```python
from build123d import *

# Parameters (mm, degrees)
SKETCH_1_R      = 1.5
EXTRUDE_1_DEPTH = 1.2
SKETCH_2_W      = 56.26507056
SKETCH_2_H      = 7.246466171
SKETCH_2_W_2    = 5.94694539
SKETCH_2_H_2    = 46.466862472
SKETCH_2_W_3    = 61.857792897
SKETCH_2_H_3    = 5.88577246
SKETCH_2_W_4    = 11.220508583
SKETCH_2_H_4    = 22.405589271
EXTRUDE_2_DEPTH = 9


with BuildPart() as part:
    # 草图1 → 凸台-拉伸1 (new body)
    with BuildSketch(Plane(origin=(0, 0, 0), x_dir=(1, 0, 0), z_dir=(0, 1, 0))):
        with BuildLine():
            Line((39.65, 36.5), (-39.65, 36.5))
            ThreePointArc((-39.65, 36.5), (-41.771320344, 35.621320344), (-42.65, 33.5))
            Line((-42.65, 33.5), (-42.65, -33.5))
            ThreePointArc((-42.65, -33.5), (-41.771320344, -35.621320344), (-39.65, -36.5))
            Line((-39.65, -36.5), (39.65, -36.5))
            ThreePointArc((39.65, -36.5), (41.771320344, -35.621320344), (42.65, -33.5))
            Line((42.65, -33.5), (42.65, 33.5))
            ThreePointArc((42.65, 33.5), (41.771320344, 35.621320344), (39.65, 36.5))
        make_face()
        with Locations(Location((39.65, -33.5, 0), (0, 0, 270))):
            Circle(SKETCH_1_R, mode=Mode.SUBTRACT)
        with Locations(Location((-39.65, -33.5, 0), (0, 0, 270))):
            Circle(SKETCH_1_R, mode=Mode.SUBTRACT)
        with Locations(Location((-39.65, 33.5, 0), (0, 0, 270))):
            Circle(SKETCH_1_R, mode=Mode.SUBTRACT)
        with Locations(Location((39.65, 33.5, 0), (0, 0, 270))):
            Circle(SKETCH_1_R, mode=Mode.SUBTRACT)
    extrude(amount=EXTRUDE_1_DEPTH)

    # 草图2 → 凸台-拉伸2 (add)
    with BuildSketch(Plane(origin=(0, 1.2, 0), x_dir=(1, 0, 0), z_dir=(0, 1, 0))):
        with Locations((3.299265125, -32.876766915)):
            Rectangle(SKETCH_2_W, SKETCH_2_H)
        with Locations((39.676527305, 1.231104757)):
            Rectangle(SKETCH_2_W_2, SKETCH_2_H_2)
        with Locations((-0.500594968, 33.55711377)):
            Rectangle(SKETCH_2_W_3, SKETCH_2_H_3)
        with Locations((-37.039745709, 3.646177151)):
            Rectangle(SKETCH_2_W_4, SKETCH_2_H_4)
    extrude(amount=EXTRUDE_2_DEPTH)


solid = part.part
```
Model file for the job. Use its own axes, mm. A direction names the side the tool comes from. Coordinates: 2 decimals unless noted, no trailing zeros. Loops run counter-clockwise (first coordinate to the right, second up) from the corner with the lowest first, then second, coordinate; pieces in that order, holes last. Notation, with made-up numbers: M 55,-14 L 93,-14 A21 ccw 93,-3 Z; hole C 1.25,36.5 d3. An arc over 180 degrees is marked long. Use CSV: the item, a comma, the result in double quotes. Start each with the question number.
1. Flat gauge pins, fed straight in: pin 1 (3 mm diameter, centred on x = 13, z = -0.5, fed in from +Y); pin 2 (6 mm diameter, centred on x = -33, y = 7.5, fed in from +Z); pin 3 (4.5 mm diameter, centred on y = 6, z = -33, fed in from -X). Where does each tip first touch, or does it go through?
2. Probe probe 1 along X at (y, z) = (0.95, -33.5); probe 2 along X at (y, z) = (4.25, -7); probe 3 along Z at (x, y) = (26, 8). List the from-to ranges inside material, lowest first. Write a range as [from, to].
3. Band-saw the part on A-A, the plane y = 3.75. List the corners of the cut face in (x, z), then the cut area to 3 significant figures.
4. Band-saw the part on D-D, the plane z = 26. List the corners of the cut face in (x, y).
5. Two-plate mould, pull along Z, no slides. Class faces 5 (the flat face through (-1, 6, -30.614)), 6 (the flat face through (-24.833, 6, 33)), 7 (the cylindrical face through (41.75, 0.59, 35.64)): pulls with the +Z half, pulls with the -Z half, needs draft (parallel to the pull), parting line crosses it, or undercut.
6. Band-saw the part on B-B, the plane z = -22. List the corners of the cut face in (x, y).
7. Tool access for faces 1 (the flat face through (3, 6, 29.254)), 2 (the flat face through (40, 6, 22.002)), 3 (the flat face through (30.428, 6, -34)), 4 (the flat face through (-37, 6, -14.849)): list every direction of +Z, -Z, +X, -X, +Y, -Y with a clear straight run to the whole face (end or side of a thin tool).
8. Band-saw the part on C-C, the plane x = -4. List the corners of the cut face in (y, z).
Entries:
1,pin 1,"stops at y = 1.2"
1,pin 2,"stops at z = 7.56"
1,pin 3,"stops at x = -31.43"
2,probe 1,"x = [-42.65, -41.15], [-38.15, 38.15], [41.15, 42.65]"
2,probe 2,"x = [-42.65, -31.43], [36.7, 42.65]"
2,probe 3,"z = [-36.5, -30.61], [29.25, 36.5]"
3,outline,"M -42.65,-14.85 L -31.43,-14.85 L -31.43,7.56 L -42.65,7.56 Z; M -31.43,-36.5 L 30.43,-36.5 L 30.43,-30.61 L -31.43,-30.61 Z; M -24.83,29.25 L 31.43,29.25 L 31.43,36.5 L -24.83,36.5 Z; M 36.7,-24.46 L 42.65,-24.46 L 42.65,22 L 36.7,22 Z"
3,area,"1,300 mm2"
4,outline,"M -42.65,0 L 42.65,0 L 42.65,1.2 L -42.65,1.2 Z"
5,face 5,"undercut"
5,face 6,"needs draft"
5,face 7,"pulls with the +Z half"
6,outline,"M -42.65,0 L 42.65,0 L 42.65,10.2 L 36.7,10.2 L 36.7,1.2 L -42.65,1.2 Z"
7,face 1,"+X, -X, +Y"
7,face 2,"+Z, +X, -X, +Y"
7,face 3,"-Z, +X, +Y"
7,face 4,"-Z, -X, +Y"
8,outline,"M 0,-36.5 L 10.2,-36.5 L 10.2,-30.61 L 1.2,-30.61 L 1.2,29.25 L 10.2,29.25 L 10.2,36.5 L 0,36.5 Z"
